The model under review builds one solid part; all positions refer to its coordinate system, in mm. Round coordinates to 2 decimals unless told otherwise and drop trailing zeros. Order: outer loops, then holes, each group sorted by start corner. A loop starts at its lowest first (then second) coordinate and runs counter-clockwise, first axis right, second up. Notation, with made-up numbers: M -28,58 L 5,58 A9 cw 5,63 Z; hole C 24,2.25 d5. An arc over 180 degrees is marked long. Answer as a JSON object with one key per item and string values. Group by question number.
1. To check wall thickness, follow probe 1 along Z at (x, y) = (30, 77); probe 2 along Z at (x, y) = (2, 51.5); probe 3 along Z at (x, y) = (37, 56). State the ranges of each line that lie inside material, in increasing order. Write a range as [from, to].
2. Clearance check with flat-ended pins moving along their axes: P1, Ø1, axis at x = -24, y = 1.5, coming from the +Z side; P2, Ø1.5, axis at x = -7.5, y = -34, coming from the -Z side; P3, Ø4, axis at y = 37, z = 20.5, coming from the -X side. State where each tip first meets the part, or that it passes through.
3. Add section C-C on y = 18. State the section outline as (x, z) points.
4. Add section B-B on x = 11. State the section outline as (y, z) points.
5. Add section A-A on z = 0. State the section outline as (x, y) points.
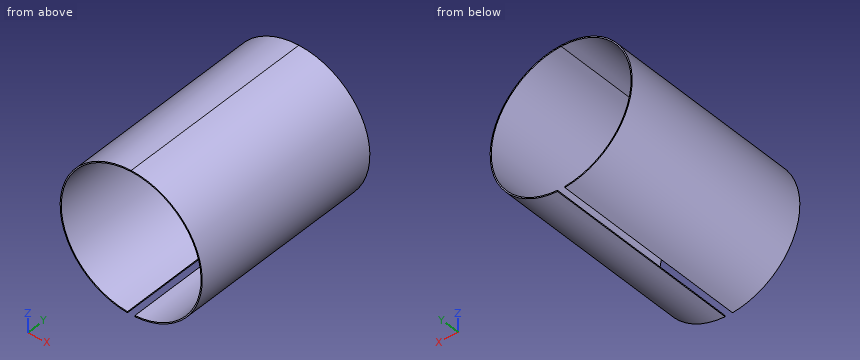
```python
from build123d import *

# Parameters (mm, degrees)
SKETCH1_R           = 62.5
SKETCH1_R_2         = 61.5
BOSS_EXTRUDE1_DEPTH = 87.5
SKETCH2_W           = 6.5
SKETCH2_H           = 1.085934022
CUT_EXTRUDE1_DEPTH  = 197.054839267


with BuildPart() as part:
    # Sketch1 → Boss-Extrude1 (new, symmetric)
    with BuildSketch(Plane(origin=(0, 0, 0), x_dir=(1, 0, 0), z_dir=(0, 1, 0))):
        with Locations(Location((0, 0, 0), (0, 0, 270))):
            Circle(SKETCH1_R)
        with Locations(Location((0, 0, 0), (0, 0, 270))):
            Circle(SKETCH1_R_2, mode=Mode.SUBTRACT)
    extrude(amount=BOSS_EXTRUDE1_DEPTH, both=True)

    # Sketch2 → Cut-Extrude1 (cut, through all)
    with BuildSketch(Plane(origin=(0, 87.5, 0), x_dir=(1, 0, 0), z_dir=(0, 1, 0))):
        with Locations((0, 61.957032989)):
            Rectangle(SKETCH2_W, SKETCH2_H)
    extrude(amount=-CUT_EXTRUDE1_DEPTH, mode=Mode.SUBTRACT)


solid = part.part
```
Recorded:
{
 "1": {"probe 1": "z = [-54.83, -53.69], [53.69, 54.83]", "probe 2": "z = [61.47, 62.47]", "probe 3": "z = [-50.37, -49.12], [49.12, 50.37]"},
 "2": {"P1": "stops at z = 57.91", "P2": "stops at z = -62.13", "P3": "stops at x = -59.7"},
 "3": {"outline": "M -3.25,-62.42 L -3.25,-61.41 A61.5 cw long 3.25,-61.41 L 3.25,-62.42 A62.5 ccw long Z"},
 "4": {"outline": "M -87.5,-61.52 L 87.5,-61.52 L 87.5,-60.51 L -87.5,-60.51 Z; M -87.5,60.51 L 87.5,60.51 L 87.5,61.52 L -87.5,61.52 Z"},
 "5": {"outline": "M -62.5,-87.5 L -61.5,-87.5 L -61.5,87.5 L -62.5,87.5 Z; M 61.5,-87.5 L 62.5,-87.5 L 62.5,87.5 L 61.5,87.5 Z"}
}
